Check sheet for the modelled part. Datum: model origin and axes. Units: mm. A direction names the side the tool comes from. Coordinates: 2 decimals unless noted, no trailing zeros. Loops run counter-clockwise (first coordinate to the right, second up) from the corner with the lowest first, then second, coordinate; pieces in that order, holes last.
```python
from build123d import *

# Parameters (mm, degrees)
BOSS_EXTRUDE1_DEPTH = 5
SKETCH2_R           = 4.9
CUT_EXTRUDE1_DEPTH  = 3.96875
CUT_EXTRUDE2_REACH  = 3.031
SKETCH3_R           = 2
FILLET1_R           = 5
CHAMFER1_SIZE       = 0.2
SKETCH5_R           = 0.15


with BuildPart() as part:
    # Sketch1 → Boss-Extrude1 (new body)
    with BuildSketch(Plane.XY):
        Polygon((7.998, 12.5), (5.998, 12.5), (5.998, 15.675), (3.498, 15.675), (3.498, 12.5), (1.15, 12.5), (1.15, 10), (2.15, 10), (2.15, 8), (1.15, 8), (1.15, 4.5), (-1.15, 4.5), (-1.15, 8), (-2.15, 8), (-2.15, 10), (-1.15, 10), (-1.15, 12.5), (-3.498, 12.5), (-3.498, 15.675), (-5.998, 15.675), (-5.998, 12.5), (-7.998, 12.5), (-7.998, -12.5), (7.998, -12.5), align=None)
    extrude(amount=BOSS_EXTRUDE1_DEPTH)

    # Sketch2 → Cut-Extrude1 (cut)
    with BuildSketch(Plane(origin=(0, 0, 0), x_dir=(-1, 0, 0), z_dir=(0, 0, -1))):
        with Locations((0, -4.5)):
            Circle(SKETCH2_R)
    extrude(amount=-CUT_EXTRUDE1_DEPTH, mode=Mode.SUBTRACT)

    # Sketch3 → Cut-Extrude2 (cut, up to next)
    with BuildSketch(Plane(origin=(0, 0, 3.96875), x_dir=(-1, 0, 0), z_dir=(0, 0, -1)), mode=Mode.PRIVATE) as cut_extrude2_sk1:
        with Locations((0, -4.5)):
            Circle(SKETCH3_R)
    cut_extrude2_tool1 = extrude(cut_extrude2_sk1.sketch, amount=-CUT_EXTRUDE2_REACH, mode=Mode.PRIVATE) & part.part
    add(cut_extrude2_tool1.solids().sort_by_distance((0, -4.5, 3.96875))[0], mode=Mode.SUBTRACT)

    # Fillet1
    fillet1_edges = [part.edges().sort_by_distance(p)[0] for p in [
        (7.998, -12.5, 2.5),
        (-7.998, -12.5, 2.5),
    ]]
    fillet(fillet1_edges, radius=FILLET1_R)

    # Chamfer1
    chamfer1_edges = [part.edges().sort_by_distance(p)[0] for p in [
        (4.9, -4.5, 0),
    ]]
    chamfer(chamfer1_edges, length=CHAMFER1_SIZE)

    # Sketch5 → Cut-Revolve1 (revolve, cut)
    with BuildSketch(Plane(origin=(0, 0, 0), x_dir=(0, 0, -1), z_dir=(1, 0, 0))):
        with Locations((-3.86875, -9.3)):
            Circle(SKETCH5_R)
    revolve(axis=Axis((0, -4.5, 5), (0, 0, -1)), mode=Mode.SUBTRACT)


solid = part.part
```
1) Scan lines: line 1 (X direction, y = -4.5, z = 1.45); line 2 (Y direction, x = 0, z = 4.6); line 3 (Y direction, x = 0, z = 1.05). Record each from-to range of solid material in increasing order.
Answer sheet:
line 1: x = -8 to -4.9, 4.9 to 8
line 2: y = -12.5 to -6.5, -2.5 to 4.5
line 3: y = -12.5 to -9.4, 0.4 to 4.5
2) Depth check by flat-ended pin: pin 1 (1.1 mm diameter, centred on x = -1.5, z = 2.5, fed in from +Y); pin 2 (1.8 mm diameter, centred on x = 0, z = 3, fed in from +Y); pin 3 (1.6 mm diameter, centred on y = 13.5, z = 3, fed in from +X); pin 4 (3.5 mm diameter, centred on x = 0, y = -4.5, fed in from +Z). Enter the tip coordinate at first touch or a pass-through.
Answer sheet:
pin 1: stops at y = 12.5
pin 2: stops at y = 4.5
pin 3: stops at x = 6
pin 4: passes through
3) Section check C-C on x = 0. Enter the section's corners in (y, z), plus the area to 3 significant figures.
Answer sheet:
outline: (-12.5, 0) - (-9.6, 0) - (-9.4, 0.2) - (-9.4, 3.76) arc R0.15 cw (long way) to (-9.19, 3.97) - (-6.5, 3.97) - (-6.5, 5) - (-12.5, 5) - close; (-2.5, 3.97) - (0.19, 3.97) arc R0.15 cw (long way) to (0.4, 3.76) - (0.4, 0.2) - (0.6, 0) - (4.5, 0) - (4.5, 5) - (-2.5, 5) - close
area: 41.9 mm2
4) Section check D-D on y = -4.5. Enter the section's corners in (x, z).
Answer sheet:
outline: (-8, 0) - (-5.1, 0) - (-4.9, 0.2) - (-4.9, 3.76) arc R0.15 cw (long way) to (-4.69, 3.97) - (-2, 3.97) - (-2, 5) - (-8, 5) - close; (2, 3.97) - (4.69, 3.97) arc R0.15 cw (long way) to (4.9, 3.76) - (4.9, 0.2) - (5.1, 0) - (8, 0) - (8, 5) - (2, 5) - close
5) Section check B-B on z = 1. Enter the section's corners in (x, y) (3 decimals).
Answer sheet:
outline: (-7.998, -7.5) arc R5 ccw to (-2.998, -12.5) - (2.998, -12.5) arc R5 ccw to (7.998, -7.5) - (7.998, 12.5) - (5.998, 12.5) - (5.998, 15.675) - (3.498, 15.675) - (3.498, 12.5) - (1.15, 12.5) - (1.15, 10) - (2.15, 10) - (2.15, 8) - (1.15, 8) - (1.15, 4.5) - (-1.15, 4.5) - (-1.15, 8) - (-2.15, 8) - (-2.15, 10) - (-1.15, 10) - (-1.15, 12.5) - (-3.498, 12.5) - (-3.498, 15.675) - (-5.998, 15.675) - (-5.998, 12.5) - (-7.998, 12.5) - close; hole circle Ø9.8 at (0, -4.5)
6) Set-up check for faces 1 (the flat face through (2.15, 9, 2)), 2 (the cylindrical face through (1.062, -9.283, 1.954)), 3 (the flat face through (-5.998, 14, 2)): record each of +Z, -Z, +X, -X, +Y, -Y from which the full face is reachable in a straight line by a thin tool's end or side.
Answer sheet:
face 1: +Z, -Z
face 2: -Z
face 3: +Z, -Z, -X, +Y
7) Section check A-A on y = 10.75. Enter the section's corners in (x, z), plus the area to 3 significant figures.
Answer sheet:
outline: (-8, 0) - (-1.15, 0) - (-1.15, 5) - (-8, 5) - close; (1.15, 0) - (8, 0) - (8, 5) - (1.15, 5) - close
area: 68.5 mm2
